Autodesk Inventor part; units mm, degrees
ref_plane "YZ Plane" through (0, 0, 0) normal (1, 0, 0) x (0, 1, 0)
ref_plane "XZ Plane" through (0, 0, 0) normal (0, 1, 0) x (-1, 0, 0)
ref_plane "XY Plane" through (0, 0, 0) normal (0, 0, 1) x (1, 0, 0)
sketch "Boceto1" plane through (0, 0, 0) normal (0, 0, 1) x (1, 0, 0)
  circle A0 centre (-35.391, 9) radius 2
  circle A1 centre (-6.391, 31.3) radius 2
  circle A2 centre (-6.391, 75.8986) radius 2
  circle A3 centre (-35.391, 75.8986) radius 2
  circle A4 centre (-35.391, 53.6) radius 2
  circle A5 centre (-6.391, 53.6) radius 2
  circle A6 centre (-6.391, 9) radius 2
  circle A7 centre (-35.391, 31.3) radius 2
  line L0 (-39.891, 8) -> (-39.891, 77)
  arc A8 (-39.891, 8) -> (-37.891, 6) centre (-37.891, 8) ccw
  line L1 (-3.891, 6) -> (-37.891, 6)
  arc A9 (-3.891, 6) -> (-1.891, 8) centre (-3.891, 8) ccw
  line L2 (-1.891, 77) -> (-1.891, 8)
  arc A10 (-1.891, 77) -> (-3.891, 79) centre (-3.891, 77) ccw
  line L3 (-37.891, 79) -> (-3.891, 79)
  arc A11 (-37.891, 79) -> (-39.891, 77) centre (-37.891, 77) ccw
  point P0 (0, 0)
  point P1 (-20.891, 10)
  dimension "d0" = 38
extrude "Extrusión1" add sketch "Boceto1" along normal blind 3
sketch "Boceto2" plane through (0, 0, 3) normal (0, 0, 1) x (1, 0, 0)
  point P0 (0, 0)
  point P1 (-35.391, 75.8986)
  point P2 (-6.391, 75.8986)
  point P3 (-6.391, 53.6)
  point P4 (-35.391, 53.6)
  point P5 (-35.391, 31.3)
  point P6 (-6.391, 31.3)
  point P7 (-35.391, 9)
  point P8 (-6.391, 9)
hole "Hole2" at (-35.391, 75.8986, 3) at (-6.391, 75.8986, 3) at (-6.391, 53.6, 3) at (-35.391, 53.6, 3) at (-35.391, 31.3, 3) at (-6.391, 31.3, 3) at (-35.391, 9, 3) at (-6.391, 9, 3) direction (0, 0, -1) diameter 4 end through all countersink diameter 8 countersink angle 90
equation "\"d17\" = Grosor"
equation "\"Radio_pliegue\" = Grosor"
equation "\"Anchura_desahogo_plegado\" = Grosor"
equation "\"Profundidad_desahogo_plegado\" = 0.5 * Grosor"
equation "\"Tamaño_destalonado\" = 4 * Grosor"
equation "\"Remanente_mínimo\" = 2 * Grosor"
equation "\"Radiodetransición\" = Radio_pliegue"
equation "\"Tamaño_de_radio_de_Jacobi\" = Radio_pliegue"
equation "\"TamañoSeparación\" = Grosor"
properties part number "Tapa"
Input: part model. Units: mm. Frame: model coordinates. Give positions to 0.01 mm unless a question says otherwise; leave off trailing zeros. Write each loop counter-clockwise with the first axis right and the second up, starting at its lowest first coordinate (ties: lowest second). Pieces come first, ordered by that corner, then holes. Notation, with made-up numbers: (35, -31) -> (74, -31) arc R16 ccw to (74, -3) -> close; hole circle Ø11 at (73.25, 6). An arc over 180 degrees is marked (long way). Use one line per item in the form item = value. Start each with the question number.
1) Draft query along X for faces 1 (the conical face through (-6.298, 33.423, 1.125)), 2 (the flat face through (-21, 79, 1)), 3 (the cylindrical face through (-2.46, 6.6, 1.48)). Return one class per face: pulls with the +X half, pulls with the -X half, needs draft (parallel to the pull), parting line crosses it, or undercut.
2) Section query B-B on z = 1.5. Count the separate pieces of the cut face and the enclosed holes in it, then the cut area to 3 significant figures.
3) Section query A-A on y = 31.3. Return the cut outline in (x, z), then the cut area to 3 significant figures.
4) Ray query, probe 1 along X at (y, z) = (9, 0.2); probe 2 along Z at (x, y) = (-8, 30); probe 3 along Z at (x, y) = (-6, 72). Return the intervals inside material, ascending. Write a range as from..to.
5) Pin query (flat end, axial travel): pin 1 (4.5 mm diameter, centred on x = -6.391, y = 31.3, fed in from +Z); pin 2 (5 mm diameter, centred on x = -35.39, y = 75.9, fed in from +Z). Return the tip coordinate at first contact, or that it passes through.
Outcome:
q1.face_1 = undercut
q1.face_2 = needs draft
q1.face_3 = pulls with the +X half
q2.separate_pieces = 1
q2.enclosed_holes = 8
q2.area = 2,610 mm^2
q3.outline = (-39.89, 0) -> (-37.39, 0) -> (-37.39, 1) -> (-39.39, 3) -> (-39.89, 3) -> close; (-33.39, 0) -> (-8.39, 0) -> (-8.39, 1) -> (-10.39, 3) -> (-31.39, 3) -> (-33.39, 1) -> close; (-4.39, 0) -> (-1.89, 0) -> (-1.89, 3) -> (-2.39, 3) -> (-4.39, 1) -> close
q3.area = 82.0 mm^2
q4.probe_1 = -39.89..-37.39, -33.39..-8.39, -4.39..-1.89
q4.probe_2 = 0..1.07
q4.probe_3 = 0..2.92
q5.pin_1 = 1.25
q5.pin_2 = 1.5
